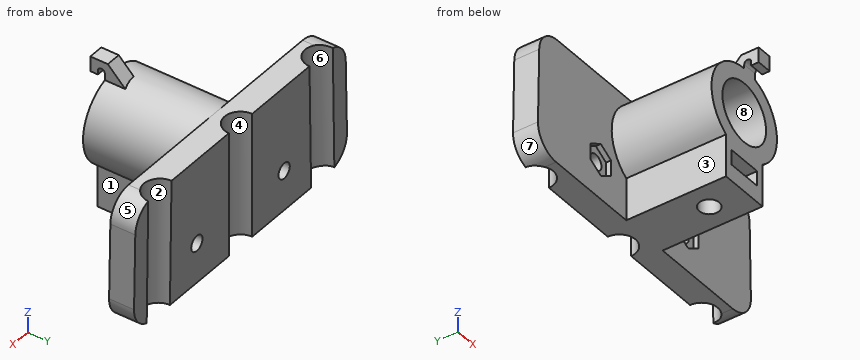
from build123d import *

# Parameters (mm, degrees)
BOSS_EXTRUDE1_DEPTH             = 5
SKETCH2_R                       = 9
SKETCH2_R_2                     = 6
BOSS_EXTRUDE2_DEPTH             = 20
SKETCH3_W                       = 10
SKETCH3_H                       = 8.516685226
BOSS_EXTRUDE3_DEPTH             = 20
SKETCH5_R                       = 3.2
CUT_EXTRUDE1_DEPTH              = 44.458424087
CIRPATTERN1_COUNT               = 2
CIRPATTERN1_ANGLE               = 1
CIRPATTERN1_THE_OTHER_WAY_COUNT = 2
CIRPATTERN1_THE_OTHER_WAY_ANGLE = 1
CUT_EXTRUDE2_REACH              = 45.458
CUT_EXTRUDE2_END_RADIUS         = 6
SKETCH6_R                       = 2
CUT_EXTRUDE2_DIRECTION_2_DEPTH  = 44.458424087
CUT_EXTRUDE3_START              = -3.3
CUT_EXTRUDE3_DEPTH              = 3
BOSS_EXTRUDE4_DEPTH             = 3
FILLET1_START                   = -20
FILLET1_DEPTH                   = 25
CUT_EXTRUDE4_DEPTH              = 1
SKETCH10_R                      = 1.55
CUT_EXTRUDE5_DEPTH              = 46.311291634


with BuildPart() as part:
    # Sketch1 → Boss-Extrude1 (new body)
    with BuildSketch(Plane(origin=(0, 0, 0), x_dir=(1, 0, 0), z_dir=(0, 1, 0))):
        Polygon((-28.820331722, 0), (-29.387661087, 25), (29.387661087, 25), (28.820331722, 0), align=None)
    extrude(amount=BOSS_EXTRUDE1_DEPTH)

    # Sketch2 → Boss-Extrude2 (add)
    with BuildSketch(Plane.XZ):
        with Locations(Location((0, -9, 0), (0, 0, 90))):
            Circle(SKETCH2_R)
        with Locations(Location((0, -9, 0), (0, 0, 270))):
            Circle(SKETCH2_R_2, mode=Mode.SUBTRACT)
    extrude(amount=BOSS_EXTRUDE2_DEPTH)

    # Sketch3 → Boss-Extrude3 (add)
    with BuildSketch(Plane.XZ):
        with Locations((0, -20.741657387)):
            Rectangle(SKETCH3_W, SKETCH3_H)
    extrude(amount=BOSS_EXTRUDE3_DEPTH)

    # Sketch5 → Cut-Extrude1 (cut, symmetric)
    with BuildSketch(Plane.XY):
        with Locations((0, 5)):
            Circle(SKETCH5_R)
    cut_extrude1 = extrude(amount=CUT_EXTRUDE1_DEPTH, both=True, mode=Mode.SUBTRACT)

    # CirPattern1: Cut-Extrude1 ×2 about axis
    cirpattern1_axis = Axis((0, 0, 1270), (0, 1, 0))
    for i in range(1, CIRPATTERN1_COUNT):
        add(cut_extrude1.rotate(cirpattern1_axis, i * CIRPATTERN1_ANGLE / (CIRPATTERN1_COUNT - 1)), mode=Mode.SUBTRACT)

    # CirPattern1 the other way: Cut-Extrude1 ×2 about axis
    cirpattern1_the_other_way_axis = Axis((0, 0, 1270), (0, -1, 0))
    for i in range(1, CIRPATTERN1_THE_OTHER_WAY_COUNT):
        add(cut_extrude1.rotate(cirpattern1_the_other_way_axis, i * CIRPATTERN1_THE_OTHER_WAY_ANGLE / (CIRPATTERN1_THE_OTHER_WAY_COUNT - 1)), mode=Mode.SUBTRACT)

    # Cut-Extrude2: up to this cylinder (the profile starts outside it)
    cut_extrude2_end = Plane(origin=(0, -13, -9), z_dir=(0, 1, 0)) * Cylinder(CUT_EXTRUDE2_END_RADIUS, 103.916, mode=Mode.PRIVATE)
    # Sketch6 → Cut-Extrude2 (cut, up to the surface)
    with BuildSketch(Plane(origin=(0, 0, -25), x_dir=(-1, 0, 0), z_dir=(0, 0, -1)), mode=Mode.PRIVATE) as cut_extrude2_sk1:
        with Locations(Location((0, -13, 0), (0, 0, 180))):
            Circle(SKETCH6_R)
    cut_extrude2_tool1 = extrude(cut_extrude2_sk1.sketch, amount=-CUT_EXTRUDE2_REACH, mode=Mode.PRIVATE) - cut_extrude2_end
    add(cut_extrude2_tool1.solids().sort_by_distance((0, -13, -25))[0], mode=Mode.SUBTRACT)

    # Sketch6 → Cut-Extrude2 direction 2 (cut)
    with BuildSketch(Plane(origin=(0, 0, -25), x_dir=(-1, 0, 0), z_dir=(0, 0, -1))):
        with Locations(Location((0, -13, 0), (0, 0, 180))):
            Circle(SKETCH6_R)
    extrude(amount=CUT_EXTRUDE2_DIRECTION_2_DEPTH, mode=Mode.SUBTRACT)

    # Sketch7 → Cut-Extrude3 (cut)
    with BuildSketch(Plane(origin=(0, 0, -25), x_dir=(-1, 0, 0), z_dir=(0, 0, -1)).offset(CUT_EXTRUDE3_START)):
        Polygon((-3.55, -15.049593456), (-3.55, -20), (3.55, -20), (3.55, -15.049593456), (3.55, -10.950406544), (0, -8.900813089), (-3.55, -10.950406544), align=None)
    extrude(amount=-CUT_EXTRUDE3_DEPTH, mode=Mode.SUBTRACT)

    # Sketch8 → Boss-Extrude4 (add)
    with BuildSketch(Plane(origin=(0, 0, 0), x_dir=(0, 0, -1), z_dir=(1, 0, 0))):
        with BuildLine():
            Line((1, -15.4), (-3, -19.4))
            Line((-3, -19.4), (-3, -22.9))
            Line((-3, -22.9), (0, -22.9))
            Line((0, -22.9), (0, -21.4))
            Line((0, -21.4), (-0.8, -21.4))
            ThreePointArc((-0.8, -21.4), (-1.5, -20.7), (-0.8, -20))
            Line((-0.8, -20), (1, -20))
            Line((1, -20), (1, -15.4))
        make_face()
    extrude(amount=BOSS_EXTRUDE4_DEPTH)

    # Fillet1: read off the stored shape, not the designer's step
    # Fillet1 outline → Fillet1 (cut)
    with BuildSketch(Plane(origin=(0, 0, 0), x_dir=(1, 0, 0), z_dir=(0, 1, 0)).offset(FILLET1_START)):
        with BuildLine():
            Line((28.820331722, 0), (28.931223357, 4.886563332))
            ThreePointArc((28.931223357, 4.886563332), (27.427708206, 1.424585105), (23.93251031, 0))
            Line((23.93251031, 0), (28.820331722, 0))
        make_face()
        with BuildLine():
            ThreePointArc((24.272907929, 25), (27.848322824, 23.495197896), (29.271620976, 19.886563332))
            Line((29.271620976, 19.886563332), (29.387661087, 25))
            Line((29.387661087, 25), (24.272907929, 25))
        make_face()
        with BuildLine():
            Line((-28.820331722, 0), (-23.93251031, 0))
            ThreePointArc((-23.93251031, 0), (-27.427708206, 1.424585105), (-28.931223357, 4.886563332))
            Line((-28.931223357, 4.886563332), (-28.820331722, 0))
        make_face()
        with BuildLine():
            ThreePointArc((-29.271620976, 19.886563332), (-27.848322824, 23.495197896), (-24.272907929, 25))
            Line((-24.272907929, 25), (-29.387661087, 25))
            Line((-29.387661087, 25), (-29.271620976, 19.886563332))
        make_face()
    extrude(amount=FILLET1_DEPTH, mode=Mode.SUBTRACT)

    # Sketch9 → Cut-Extrude4 (cut)
    with BuildSketch(Plane.XZ):
        Polygon((12, -20.233161507), (14.8, -18.616580754), (14.8, -15.383419246), (12, -13.766838493), (9.2, -15.383419246), (9.2, -18.616580754), align=None)
    cut_extrude4 = extrude(amount=-CUT_EXTRUDE4_DEPTH, mode=Mode.SUBTRACT)

    # Sketch10 → Cut-Extrude5 (cut, through all)
    with BuildSketch(Plane.XZ.offset(-1)):
        with Locations(Location((12, -17, 0), (0, 0, 270))):
            Circle(SKETCH10_R)
    cut_extrude5 = extrude(amount=-CUT_EXTRUDE5_DEPTH, mode=Mode.SUBTRACT)

    # Mirror1: Cut-Extrude4, Cut-Extrude5 across plane
    add(cut_extrude4.mirror(Plane(origin=(0, 0, 0), x_dir=(0, 0, 1), z_dir=(1, 0, 0))), mode=Mode.SUBTRACT)
    add(cut_extrude5.mirror(Plane(origin=(0, 0, 0), x_dir=(0, 0, 1), z_dir=(1, 0, 0))), mode=Mode.SUBTRACT)


solid = part.part
Could you check a few things on this model? Use its own coordinates, in mm. Face numbers are marked on the shaded views. A direction names the side the tool comes from. Coordinates: 2 decimals unless noted, no trailing zeros. Order: outer loops, then holes, each group sorted by start corner. A loop starts at its lowest first (then second) coordinate and runs counter-clockwise, first axis right, second up.
Q1. Please list where these lines run through material, in increasing order: L1, parallel to X at y = -13, z = -23; L2, parallel to X at y = 2.4, z = -17; L3, parallel to X at y = 4.1, z = -17.
Q2. Which directions (+Z, -Z, +X, -X, +Y, -Y) give clear straight access to the entire face, cutting with the end or side of a thin tool? Please do the marked faces 1, 2, 3 and 4.
Q3. Will these pins go through, and if not, where does the flat tip stop? pin 1 (1 mm diameter, centred on x = -23.5, z = -1.5, fed in from -Y); pin 2 (3.5 mm diameter, centred on x = -1.5, y = -15, fed in from +Z); pin 3 (0.5 mm diameter, centred on y = 0.5, z = -17.5, fed in from -X); pin 4 (3.5 mm diameter, centred on x = 12, z = -17, fed in from +Y).
Q4. Suppose I cut it at C-C on y = -20.7. Please give me the cut outline in (x, z).
Q5. Thinking about a two-plate mould opening in X: for the marked faces 5, 6, 7 and 8, which applies, released by +X, released by -X, zero draft, split by the parting line, or undercut?
Q6. Suppose I cut it at D-D on x = -18. Please give me the cut outline in (y, z), and give its area (3 significant figures).
Q7. Suppose I cut it at A-A on y = -9.75. Please give me the cut outline in (x, z).
Q8. Suppose I cut it at B-B on x = 7. Please give me the cut outline in (y, z).
Answer:
1. L1: x = -5 to -2, 2 to 5
1. L2: x = -29.21 to -24.33, -20.6 to -13.55, -10.45 to -1.87, 1.87 to 10.45, 13.55 to 20.6, 24.33 to 29.21
1. L3: x = -29.21 to -25.54, -19.39 to -13.55, -10.45 to -3.07, 3.07 to 10.45, 13.55 to 19.39, 25.54 to 29.21
2. face 1: -Z, +X, -Y
2. face 2: +Y
2. face 3: -Z, -X, -Y
2. face 4: +Z, -Z, +Y
3. pin 1: stops at y = 0
3. pin 2: stops at z = 0
3. pin 3: stops at x = -29.22
3. pin 4: stops at y = 5
4. outline: (0, 1.5) - (3, 1.5) - (3, 3) - (0, 3) - close
5. face 5: released by +X
5. face 6: undercut
5. face 7: released by -X
5. face 8: undercut
6. outline: (0, -25) - (5, -25) - (5, 0) - (0, 0) - close
6. area: 125 mm2
7. outline: (-5, -25) - (5, -25) - (5, -16.48) arc R9 ccw (long way) to (-5, -16.48) - close; hole circle Ø12 at (0, -9); hole (-1.47, -21.7) - (1.47, -21.7) - (1.47, -18.7) - (-1.47, -18.7) - close
8. outline: (-20, -14.66) - (0, -14.66) - (0, -25) - (5, -25) - (5, 0) - (0, 0) - (0, -3.34) - (-20, -3.34) - close
